from build123d import *

# Parameters (mm, degrees)
SKETCH_1_W          = 35
SKETCH_1_H          = 10
EXTRUDE_1_DEPTH     = 2
SKETCH_3_W          = 35
SKETCH_3_H          = 2
EXTRUDE_2_DEPTH     = 2
SKETCH_3_3_W        = 35
SKETCH_3_3_H        = 4.7
EXTRUDE_3_DEPTH     = 4
SKETCH_4_R          = 0.35
CUT_EXTRUDE_1_DEPTH = 20.163767897


with BuildPart() as part:
    # 草图1 → 凸台-拉伸1 (new body)
    with BuildSketch(Plane.XY):
        Rectangle(SKETCH_1_W, SKETCH_1_H)
    extrude(amount=EXTRUDE_1_DEPTH)

    # 草图3 → 凸台-拉伸2 (add)
    with BuildSketch(Plane.XY.offset(2)):
        with Locations((0, 4)):
            Rectangle(SKETCH_3_W, SKETCH_3_H)
    extrude(amount=EXTRUDE_2_DEPTH)

    # 草图3<3> → 凸台-拉伸3 (add)
    with BuildSketch(Plane.XY.offset(2)):
        with Locations((0, -2.65)):
            Rectangle(SKETCH_3_3_W, SKETCH_3_3_H)
    extrude(amount=EXTRUDE_3_DEPTH)

    # 草图4 → 切除-拉伸1 (cut, through all)
    with BuildSketch(Plane.XY.offset(6)):
        with Locations((15.5, -3)):
            Circle(SKETCH_4_R)
        with Locations((-15.5, -3)):
            Circle(SKETCH_4_R)
    extrude(amount=-CUT_EXTRUDE_1_DEPTH, mode=Mode.SUBTRACT)


solid = part.part
CAD build for the part. Positions are in the model's coordinates, mm. A direction names the side the tool comes from. Give positions to 0.01 mm unless a question says otherwise; leave off trailing zeros. Order: outer loops, then holes, each group sorted by start corner. A loop starts at its lowest first (then second) coordinate and runs counter-clockwise, first axis right, second up. Notation, with made-up numbers: (47, 14) - (59, 14) arc R18 ccw to (59, 37) - close; hole circle Ø10 at (-7, 78). An arc over 180 degrees is marked (long way). Answer in a Markdown table with one row per item.
1. Pull direction Y, two halves, no side cores. Call faces 1 (the flat face through (0, 1, 2)), 2 (the flat face through (0, -5, 3)), 3 (the flat face through (0, 0, 0)): pulls with the +Y half, pulls with the -Y half, needs draft (parallel to the pull), parting line crosses it, or undercut.
Data:
| item | result |
|---|---|
| face 1 | undercut |
| face 2 | pulls with the -Y half |
| face 3 | needs draft |
2. Saw through at D-D, the plane x = 10. Give the cut face in (y, z).
Data:
| item | result |
|---|---|
| outline | (-5, 0) - (5, 0) - (5, 4) - (3, 4) - (3, 2) - (-0.3, 2) - (-0.3, 6) - (-5, 6) - close |
3. Saw through at B-B, the plane y = -3. Give the cut face in (x, z).
Data:
| item | result |
|---|---|
| outline | (-17.5, 0) - (-15.85, 0) - (-15.85, 6) - (-17.5, 6) - close; (-15.15, 0) - (15.15, 0) - (15.15, 6) - (-15.15, 6) - close; (15.85, 0) - (17.5, 0) - (17.5, 6) - (15.85, 6) - close |
4. Saw through at C-C, the plane x = 15.5. Give the cut face in (y, z).
Data:
| item | result |
|---|---|
| outline | (-5, 0) - (-3.35, 0) - (-3.35, 6) - (-5, 6) - close; (-2.65, 0) - (5, 0) - (5, 4) - (3, 4) - (3, 2) - (-0.3, 2) - (-0.3, 6) - (-2.65, 6) - close |
5. Flat gauge pins, fed straight in: pin 1 (2 mm diameter, centred on x = 4.5, y = 4.5, fed in from +Z); pin 2 (1 mm diameter, centred on x = -8.5, y = 1.5, fed in from +Z). Where does each tip first touch, or does it go through?
Data:
| item | result |
|---|---|
| pin 1 | stops at z = 4 |
| pin 2 | stops at z = 2 |
6. Tool access for faces 4 (the flat face through (0, -3, 6)), 5 (the flat face through (0, 4, 4)), 6 (the flat face through (0, -0.3, 4)): list every direction of +Z, -Z, +X, -X, +Y, -Y with a clear straight run to the whole face (end or side of a thin tool).
Data:
| item | result |
|---|---|
| face 4 | +Z, +X, -X, +Y, -Y |
| face 5 | +Z, +X, -X, +Y |
| face 6 | +Z, +X, -X |
7. Saw through at A-A, the plane z = 3.6. Give the cut face in (x, y).
Data:
| item | result |
|---|---|
| outline | (-17.5, -5) - (17.5, -5) - (17.5, -0.3) - (-17.5, -0.3) - close; (-17.5, 3) - (17.5, 3) - (17.5, 5) - (-17.5, 5) - close; hole circle Ø0.7 at (-15.5, -3); hole circle Ø0.7 at (15.5, -3) |
8. Probe probe 1 along Y at (x, z) = (15.5, 2.9); probe 2 along Y at (x, z) = (8, 3.4); probe 3 along Z at (x, y) = (10, 4). List the from-to ranges inside material, lowest first. Write a range as [from, to].
Data:
| item | result |
|---|---|
| probe 1 | y = [-5, -3.35], [-2.65, -0.3], [3, 5] |
| probe 2 | y = [-5, -0.3], [3, 5] |
| probe 3 | z = [0, 4] |
